from build123d import *

# Parameters (mm, degrees)
F0_W           = 355.6
F0_H           = 152.4
F1_DEPTH       = 12.7
F3_DEPTH       = 12.701
F5_D           = 2.54
F5_CSINK_D     = 6.604
F5_CSINK_ANGLE = 90


with BuildPart() as f1:
    # F0 (on Top) → F1 (new body)
    with BuildSketch(Plane.XY):
        Rectangle(F0_W, F0_H)
    extrude(amount=F1_DEPTH)

    # F2 (on face) → F3 (cut, through all)
    with BuildSketch(Plane.XY.offset(12.7)):
        with BuildLine():
            Line((120.65, 25.4), (-146.05, 25.4))
            ThreePointArc((-146.05, 25.4), (-150.540128, 23.540128), (-152.4, 19.05))
            Line((-152.4, 19.05), (-152.4, -19.05))
            ThreePointArc((-152.4, -19.05), (-150.540128, -23.540128), (-146.05, -25.4))
            Line((-146.05, -25.4), (120.65, -25.4))
            ThreePointArc((120.65, -25.4), (125.140128, -23.540128), (127, -19.05))
            Line((127, -19.05), (127, 19.05))
            ThreePointArc((127, 19.05), (125.140128, 23.540128), (120.65, 25.4))
        make_face()
    extrude(amount=-F3_DEPTH, mode=Mode.SUBTRACT)

    # F5 (through all)
    with Locations(Plane(origin=(0, 0, 0), x_dir=(1, 0, 0), z_dir=(0, 0, -1))):
        with Locations((-152.4, 69.85), (-50.8, 69.85), (50.8, 69.85), (152.4, 69.85), (152.4, -69.85), (50.8, -69.85), (-50.8, -69.85), (-152.4, -69.85)):
            CounterSinkHole(F5_D / 2, F5_CSINK_D / 2, counter_sink_angle=F5_CSINK_ANGLE)


solid = f1.part
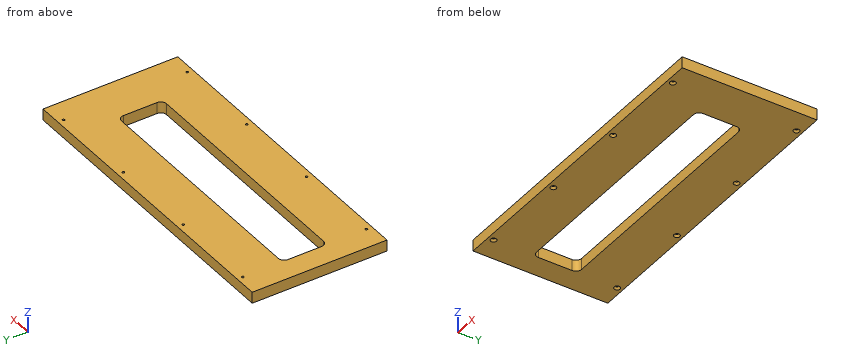
Geometry: final body of the model. Coordinates: model frame, mm. Give positions to 0.01 mm unless a question says otherwise; leave off trailing zeros. Write each loop counter-clockwise with the first axis right and the second up, starting at its lowest first coordinate (ties: lowest second). Pieces come first, ordered by that corner, then holes. Notation, with made-up numbers: (36, -23.75) - (92, -23.75) arc R34 ccw to (92, 13.25) - close; hole circle Ø8 at (36.5, 27.25). An arc over 180 degrees is marked (long way). Return JSON: item names as keys, results as strings. Group by question number.
1) Section B-B on y = 3. Return the cut outline in (x, z), plus the area to 3 significant figures.
2) Section C-C on x = -100. Return the cut outline in (y, z).
3) First-contact query: P1, Ø3, axis at x = 50.8, y = -69.85, coming from the -Z side; P2, Ø3.5, axis at x = -152.4, y = -69.85, coming from the +Z side. Flat tips, straight axial feed; report the tip coordinate or a pass-through.
4) Section A-A on z = 8.25. State how many separate pieces and enclosed holes the cut face has, plus the area to 3 significant figures.
5) Line query: line 1 (X direction, y = 69.85, z = 9); line 2 (Y direction, x = -50.8, z = 6.5); line 3 (Y direction, x = 152.4, z = 5.75). Output: solid intervals per line, ascending.
Filled in:
{
 "1": {"outline": "(-177.8, 0) - (-152.4, 0) - (-152.4, 12.7) - (-177.8, 12.7) - close; (127, 0) - (177.8, 0) - (177.8, 12.7) - (127, 12.7) - close", "area": "968 mm^2"},
 "2": {"outline": "(-76.2, 0) - (-25.4, 0) - (-25.4, 12.7) - (-76.2, 12.7) - close; (25.4, 0) - (76.2, 0) - (76.2, 12.7) - (25.4, 12.7) - close"},
 "3": {"P1": "stops at z = 1.8", "P2": "stops at z = 12.7"},
 "4": {"separate pieces": "1", "enclosed holes": "9", "area": "40,000 mm^2"},
 "5": {"line 1": "x = -177.8 to -153.67, -151.13 to -52.07, -49.53 to 49.53, 52.07 to 151.13, 153.67 to 177.8", "line 2": "y = -76.2 to -71.12, -68.58 to -25.4, 25.4 to 68.58, 71.12 to 76.2", "line 3": "y = -76.2 to -71.12, -68.58 to 68.58, 71.12 to 76.2"}
}
